Read the model definition and answer for the solid it produces. Units are mm, in the model's axes. A direction names the side the tool comes from. Coordinates: 2 decimals unless noted, no trailing zeros. Loops run counter-clockwise (first coordinate to the right, second up) from the corner with the lowest first, then second, coordinate; pieces in that order, holes last. Notation, with made-up numbers: M 16.5,39.25 L 38.5,39.25 A23 ccw 38.5,51.25 Z; hole C 5.5,89.5 d8. An arc over 180 degrees is marked long. One line per item, written item: value. Start each with the question number.
1. The part is cut by section B-B (y = 39.5). Write down the section's boundary in (x, z).
2. Determine the mould class of faces 1 (the face through (-20.58, -56.36, 0.04)), 2 (the face through (0, 14.35, 0)), 3 (the face through (-15, 10, -2.5)), 4 (the face through (8.59, 45.13, 0.04)) for opening direction Y: +Y half, -Y half, draft (parallel to the pull), parting line (faces both ways), or undercut.
3. For faces 5 (the face through (-38.517, 46.005, 0.035)), 6 (the face through (-12.38, 7.26, 0.04)), 7 (the face through (10.884, -19.352, 2.254)), determine the directions among +Z, -Z, +X, -X, +Y, -Y from which every point of the face is accessible in a straight line to the end or side of a thin tool.
4. Consider probe 1 along X at (y, z) = (8.5, -1.6); probe 2 along Y at (x, z) = (1, 2.35); probe 3 along Y at (x, z) = (12, -1.05). Determine where each line is inside the solid, lowest interval first.
5. The part is cut by section C-C (x = 30). Write down the section's boundary in (y, z).
6. The part is cut by section A-A (x = -30). Write down the section's boundary in (y, z).
7. Flat-ended cylindrical pins translate along their axes: pin 1 (2.5 mm diameter, centred on x = 1, z = 0, fed in from -Y); pin 2 (1 mm diameter, centred on x = 23, z = -1.5, fed in from -Y). Find the tip coordinate at first contact, or state that the pin passes through.
```python
from build123d import *

# Parameters (mm, degrees)
BOSS_EXTRUDE1_DEPTH = 2.5
FILLET1_R           = 10
CUT_EXTRUDE1_DEPTH  = 0.5


with BuildPart() as part:
    # Sketch1 → Boss-Extrude1 (new, symmetric)
    with BuildSketch(Plane.XY):
        with BuildLine():
            ThreePointArc((-34.426436475, 49.140822863), (-38.572797774, 45.958016405), (-42.426406871, 42.426406871))
            ThreePointArc((-42.426406871, 42.426406871), (-26.29235792, 40.654943242), (-22.609103215, 24.847373735))
            ThreePointArc((-22.609103215, 24.847373735), (-43.353983992, -14.099744614), (-25.343982725, -54.38457998))
            ThreePointArc((-25.343982725, -54.38457998), (-20.514410827, -56.38403097), (-15.529142706, -57.955549577))
            ThreePointArc((-15.529142706, -57.955549577), (-22.062034677, -43.097321505), (-10.213905264, -32.003744609))
            ThreePointArc((-10.213905264, -32.003744609), (33.887729018, -30.495779185), (59.7704192, 5.243757117))
            ThreePointArc((59.7704192, 5.243757117), (59.087208601, 10.426014565), (57.955549577, 15.529142706))
            ThreePointArc((57.955549577, 15.529142706), (48.354392597, 2.442378263), (32.82300848, 7.156370874))
            ThreePointArc((32.82300848, 7.156370874), (9.466254973, 44.595523799), (-34.426436475, 49.140822863))
        make_face()
        with BuildLine():
            Line((-15.848264889, -1.25), (-9.006664199, -13.1))
            ThreePointArc((-9.006664199, -13.1), (-8.895018703, -13.516666667), (-9.006664199, -13.933333333))
            ThreePointArc((-9.006664199, -13.933333333), (-8.70164303, -15.071687836), (-7.563288526, -14.766666667))
            ThreePointArc((-7.563288526, -14.766666667), (-7.258267357, -14.461645497), (-6.84160069, -14.35))
            Line((-6.84160069, -14.35), (6.84160069, -14.35))
            ThreePointArc((6.84160069, -14.35), (7.258267357, -14.461645497), (7.563288526, -14.766666667))
            ThreePointArc((7.563288526, -14.766666667), (8.70164303, -15.071687836), (9.006664199, -13.933333333))
            ThreePointArc((9.006664199, -13.933333333), (8.895018703, -13.516666667), (9.006664199, -13.1))
            Line((9.006664199, -13.1), (15.848264889, -1.25))
            ThreePointArc((15.848264889, -1.25), (16.153286059, -0.94497883), (16.569952726, -0.833333333))
            ThreePointArc((16.569952726, -0.833333333), (17.403286059, 0), (16.569952726, 0.833333333))
            ThreePointArc((16.569952726, 0.833333333), (16.153286059, 0.94497883), (15.848264889, 1.25))
            Line((15.848264889, 1.25), (9.006664199, 13.1))
            ThreePointArc((9.006664199, 13.1), (8.895018703, 13.516666667), (9.006664199, 13.933333333))
            ThreePointArc((9.006664199, 13.933333333), (8.70164303, 15.071687836), (7.563288526, 14.766666667))
            ThreePointArc((7.563288526, 14.766666667), (7.258267357, 14.461645497), (6.84160069, 14.35))
            Line((6.84160069, 14.35), (-6.84160069, 14.35))
            ThreePointArc((-6.84160069, 14.35), (-7.258267357, 14.461645497), (-7.563288526, 14.766666667))
            ThreePointArc((-7.563288526, 14.766666667), (-8.70164303, 15.071687836), (-9.006664199, 13.933333333))
            ThreePointArc((-9.006664199, 13.933333333), (-8.895018703, 13.516666667), (-9.006664199, 13.1))
            Line((-9.006664199, 13.1), (-15.848264889, 1.25))
            ThreePointArc((-15.848264889, 1.25), (-16.153286059, 0.94497883), (-16.569952726, 0.833333333))
            ThreePointArc((-16.569952726, 0.833333333), (-17.403286059, 0), (-16.569952726, -0.833333333))
            ThreePointArc((-16.569952726, -0.833333333), (-16.153286059, -0.94497883), (-15.848264889, -1.25))
        make_face(mode=Mode.SUBTRACT)
    extrude(amount=BOSS_EXTRUDE1_DEPTH, both=True)

    # Fillet1
    fillet1_edges = [part.edges().sort_by_distance(p)[0] for p in [
        (32.82300848, 7.156370874, 0),
        (-10.213905264, -32.003744609, 0),
        (-22.609103215, 24.847373735, 0),
    ]]
    fillet(fillet1_edges, radius=FILLET1_R)

    # Sketch2 → Cut-Extrude1 (cut)
    with BuildSketch(Plane.XY.offset(2.5)):
        Polygon((8.66814938, -14.513675135), (13.66814938, -23.173929172), (13.235136679, -23.423929172), (8.235136679, -14.763675135), align=None)
        Polygon((16.834018905, -0.25029747), (16.834004031, 0.249702529), (26.834004027, 0.25), (26.8340189, -0.25), align=None)
        Polygon((8.564068882, 14.452995813), (8.131041308, 14.702970051), (13.130526065, 23.363521544), (13.563553639, 23.113547307), align=None)
    extrude(amount=-CUT_EXTRUDE1_DEPTH, mode=Mode.SUBTRACT)


solid = part.part
```
Answer block:
1. outline: M -25.13,-2.5 L 16.27,-2.5 L 16.27,2.5 L -25.13,2.5 Z
2. face 1: -Y half
2. face 2: undercut
2. face 3: draft
2. face 4: +Y half
3. face 5: +Z, -Z, -X, +Y
3. face 6: +Z, -Z
3. face 7: +Z
4. probe 1: x = -37.09 to -11.66, 11.66 to 32.9, 55.93 to 59.39
4. probe 2: y = -35.52 to -14.35, 14.35 to 48.83
4. probe 3: y = -36.35 to -7.92, 7.92 to 42.9
5. outline: M -32.36,-2.5 L 19.34,-2.5 L 19.34,2.5 L -32.36,2.5 Z
6. outline: M -49.96,-2.5 L 18.3,-2.5 L 18.3,2.5 L -49.96,2.5 Z; M 43.02,-2.5 L 50.54,-2.5 L 50.54,2.5 L 43.02,2.5 Z
7. pin 1: stops at y = -35.73
7. pin 2: stops at y = -34.88
